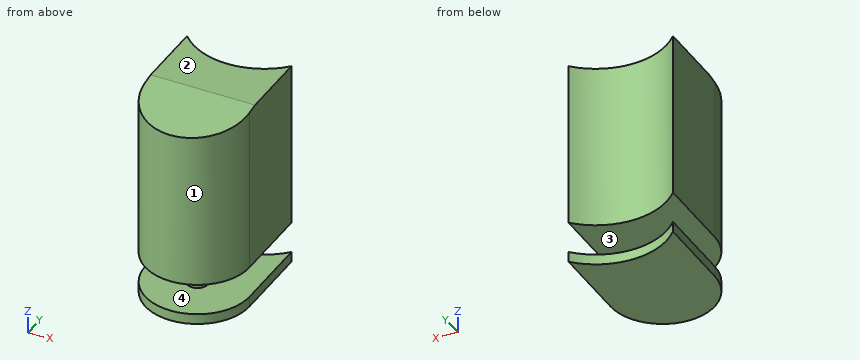
Autodesk Inventor part; units mm, degrees
ref_plane "YZ Plane" through (0, 0, 0) normal (1, 0, 0) x (0, 1, 0)
ref_plane "XZ Plane" through (0, 0, 0) normal (0, 1, 0) x (-1, 0, 0)
ref_plane "XY Plane" through (0, 0, 0) normal (0, 0, 1) x (1, 0, 0)
sketch "Sketch1" plane through (0, 0, 0) normal (0, 0, 1) x (1, 0, 0)
  line L0 (0, 15.9441) -> (0, -15.9441) construction
  line L1 (11.6084, 0) -> (-11.6084, 0) construction
  line L2 (50, 162.8204) -> (50, 85.9072)
  line L3 (50, 85.9072) -> (-50, 85.9072)
  line L4 (-50, 85.9072) -> (-50, 162.8204)
  circle A0 centre (0, 85.9072) radius 50
  arc A1 (-50, 162.8204) -> (50, 162.8204) centre (0, 208.9072) ccw
  point P0 (0, 0)
  point P1 (0, 0)
  point P2 (0, 165.9072)
  dimension "d5" = 100
  dimension "d7" = 136
  dimension "d8" = 123
extrude "Extrusion1" add sketch "Sketch1" along normal blind 200
sketch "Sketch2" plane through (50, 85.9072, 0) normal (1, 0, 0) x (0, 0, -1)
  line L0 (-200, 10) -> (-186.1081, -68.7846)
  line L1 (-200, 10) -> (-200, -68.7846)
  line L2 (-200, -68.7846) -> (-186.1081, -68.7846)
  point P0 (0, -85.9072)
extrude "Extrusion2" cut sketch "Sketch2" against normal through all
sketch "Sketch3" plane through (50, 85.9072, 0) normal (1, 0, 0) x (0, 0, -1)
  line L0 (-40, 89.4296) -> (-10, 89.4296)
  line L1 (-10, 89.4296) -> (-10, -119.3946)
  line L2 (-10, -119.3946) -> (-40, -119.3946)
  line L3 (-40, -119.3946) -> (-40, 89.4296)
  line L4 (0, -50) -> (0, 0)
  line L5 (0, 76.9131) -> (-200, 76.9131)
  point P0 (0, -85.9072)
  dimension "d9" = 30
  dimension "d10" = 10
extrude "Extrusion3" cut sketch "Sketch3" against normal through all
sketch "Sketch4" plane through (50, 85.9072, 10) normal (0, 0, 1) x (1, 0, 0)
  arc A0 (-100, 0) -> (0, 0) centre (-50, 0) ccw
  circle A1 centre (-50, 0) radius 10
  point P0 (-50, -85.9072)
extrude "Extrusion4" add sketch "Sketch4" along normal blind 30
properties part number "CANH TAY 1"
Source: CAD feature listing. Evaluate the final solid. Frame: model axes, mm. Face numbers are marked on the shaded views. Give positions to 0.01 mm unless a question says otherwise; leave off trailing zeros. Order: outer loops, then holes, each group sorted by start corner. A loop starts at its lowest first (then second) coordinate and runs counter-clockwise, first axis right, second up. Notation, with made-up numbers: (52.25, -5.5) -> (91.25, -5.5) arc R15 ccw to (91.25, 22.5) -> close; hole circle Ø6 at (58.25, 50.5). An arc over 180 degrees is marked (long way). Use a Markdown table: item, result.
Q1. First-contact query: P1, Ø10, axis at y = 61, z = 153.5, coming from the -X side; P2, Ø12, axis at x = 18.5, z = 93.5, coming from the +Y side; P3, Ø2, axis at y = 50.5, z = 67, coming from the +X side. Flat tips, straight axial feed; report the tip coordinate or a pass-through.
A:
| item | result |
|---|---|
| P1 | x = -45.87 |
| P2 | y = 145.47 |
| P3 | x = 36.28 |
Q2. Section B-B (x = 0). Return the cut outline in (y, z), and give its area (3 significant figures).
A:
| item | result |
|---|---|
| outline | (35.91, 0) -> (140.91, 0) -> (140.91, 10) -> (95.91, 10) -> (95.91, 40) -> (140.91, 40) -> (140.91, 200) -> (95.91, 200) -> (35.91, 189.42) -> (35.91, 40) -> (75.91, 40) -> (75.91, 10) -> (35.91, 10) -> close |
| area | 18,100 mm^2 |
Q3. Material intervals for line 1 (Z direction, x = -10, y = 115); line 2 (Y direction, x = -1, z = 161); line 3 (X direction, y = 150, z = 84.5), sorted ascending. Write a range as [from, to].
A:
| item | result |
|---|---|
| line 1 | [0, 10], [40, 200] |
| line 2 | [35.92, 140.91] |
| line 3 | [-50, -33.97], [33.97, 50] |
Q4. Section D-D (x = 24). Return the cut outline in (y, z).
A:
| item | result |
|---|---|
| outline | (42.04, 0) -> (145.28, 0) -> (145.28, 10) -> (42.04, 10) -> close; (42.04, 40) -> (145.28, 40) -> (145.28, 200) -> (95.91, 200) -> (42.04, 190.5) -> close |
Q5. Section A-A (y = 101.5). Return the cut outline in (x, z), and give its area (3 significant figures).
A:
| item | result |
|---|---|
| outline | (-50, 0) -> (50, 0) -> (50, 10) -> (-50, 10) -> close; (-50, 40) -> (50, 40) -> (50, 200) -> (-50, 200) -> close |
| area | 17,000 mm^2 |
Q6. Section C-C (z = 184.5). Return the cut outline in (x, y).
A:
| item | result |
|---|---|
| outline | (-50, 85.91) arc R50 ccw to (50, 85.91) -> (50, 162.82) arc R68 cw to (-50, 162.82) -> close |
Q7. Pull-direction query (Z, two-part tool) for the marked faces 1, 2, 3 and 4; classes: +Z half, -Z half, draft (parallel to the pull), parting line (faces both ways), or undercut.
A:
| item | result |
|---|---|
| face 1 | draft |
| face 2 | +Z half |
| face 3 | undercut |
| face 4 | undercut |
